Read the model definition and answer for the solid it produces. Units are mm, in the model's axes. Face numbers are marked on the shaded views. A direction names the side the tool comes from. Coordinates: 2 decimals unless noted, no trailing zeros. Order: outer loops, then holes, each group sorted by start corner. A loop starts at its lowest first (then second) coordinate and runs counter-clockwise, first axis right, second up. Notation, with made-up numbers: (10.5, -30.75) -> (54.5, -30.75) arc R20 cw to (54.5, -18.75) -> close; hole circle Ø5 at (17.5, 11). An arc over 180 degrees is marked (long way). Use CSV: the item, a comma, the result in double quotes.
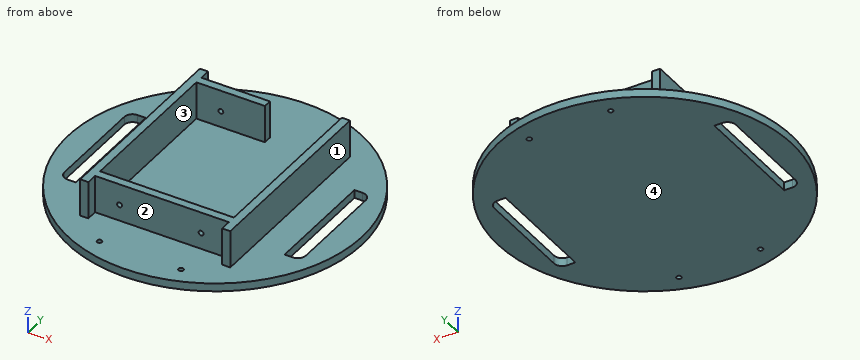
```python
from build123d import *

# Parameters (mm, degrees)
SKETCH_1_R          = 90
EXTRUDE_1_DEPTH     = 5
CUT_EXTRUDE_1_DEPTH = 128.377392029
SKETCH_2_R          = 1.5
CUT_EXTRUDE_2_DEPTH = 128.377392029
SKETCH_4_W          = 5
SKETCH_4_H          = 120
EXTRUDE_2_DEPTH     = 23
SKETCH_5_W          = 82
SKETCH_5_H          = 5
SKETCH_5_W_2        = 42
EXTRUDE_3_DEPTH     = 23
SKETCH_6_R          = 1.5
CUT_EXTRUDE_3_DEPTH = 172.477585999


with BuildPart() as part:
    # 草圖1 → 填料-伸長1 (new body)
    with BuildSketch(Plane.XY):
        Circle(SKETCH_1_R)
    extrude(amount=EXTRUDE_1_DEPTH)

    # 草圖3 → 除料-伸長1 (cut, through all)
    with BuildSketch(Plane.XY.offset(5)):
        with BuildLine():
            ThreePointArc((-69, -35), (-72.535533906, -33.535533906), (-74, -30))
            Line((-74, -30), (-74, 30))
            ThreePointArc((-74, 30), (-72.535533906, 33.535533906), (-69, 35))
            Line((-69, 35), (-64, 35))
            Line((-64, 35), (-64, -35))
            Line((-64, -35), (-69, -35))
        make_face()
        with BuildLine():
            Line((64, 35), (64, -35))
            Line((64, -35), (69, -35))
            ThreePointArc((69, -35), (72.535533906, -33.535533906), (74, -30))
            Line((74, -30), (74, 30))
            ThreePointArc((74, 30), (72.535533906, 33.535533906), (69, 35))
            Line((69, 35), (64, 35))
        make_face()
    extrude(amount=-CUT_EXTRUDE_1_DEPTH, mode=Mode.SUBTRACT)

    # 草圖2 → 除料-伸長2 (cut, through all)
    with BuildSketch(Plane.XY.offset(5)):
        with Locations((-25, 75)):
            Circle(SKETCH_2_R)
        with Locations(Location((-25, -75, 0), (0, 0, 180))):
            Circle(SKETCH_2_R)
        with Locations(Location((25, 75, 0), (0, 0, 180))):
            Circle(SKETCH_2_R)
        with Locations((25, -75)):
            Circle(SKETCH_2_R)
    extrude(amount=-CUT_EXTRUDE_2_DEPTH, mode=Mode.SUBTRACT)

    # 草圖4 → 填料-伸長2 (add)
    with BuildSketch(Plane.XY.offset(5)):
        with Locations((-43.5, 0)):
            Rectangle(SKETCH_4_W, SKETCH_4_H)
        with Locations((43.5, 0)):
            Rectangle(SKETCH_4_W, SKETCH_4_H)
    extrude(amount=EXTRUDE_2_DEPTH)

    # 草圖5 → 填料-伸長3 (add)
    with BuildSketch(Plane.XY.offset(5)):
        with Locations((0, -50.75)):
            Rectangle(SKETCH_5_W, SKETCH_5_H)
        with Locations((-20, 50.75)):
            Rectangle(SKETCH_5_W_2, SKETCH_5_H)
    extrude(amount=EXTRUDE_3_DEPTH)

    # 草圖6 → 除料-伸長3 (cut, through all)
    with BuildSketch(Plane(origin=(0, -53.25, 0), x_dir=(-1, 0, 0), z_dir=(0, -1, 0))):
        with Locations(Location((26, -15, 0), (0, 0, 90))):
            Circle(SKETCH_6_R)
        with Locations(Location((-24, -15, 0), (0, 0, 180))):
            Circle(SKETCH_6_R)
    extrude(amount=-CUT_EXTRUDE_3_DEPTH, mode=Mode.SUBTRACT)


solid = part.part
```
Item 1: Find section D-D, the plane x = -54. Give the vertices of the cut face in (y, z).
Return value:
outline,"(-72, 0) -> (72, 0) -> (72, 5) -> (-72, 5) -> close"
Item 2: A tool of negligible diameter and unlimited length cuts with its end or side. For the marked faces 1, 2, 3 and 4, from which of +Z, -Z, +X, -X, +Y, -Y can it reach the whole face along a straight path? Write none if from no direction.
Return value:
face 1,"+Z, +X, +Y, -Y"
face 2,"+Z, -Y"
face 3,"+Z"
face 4,"-Z, +X, -X, +Y, -Y"
Item 3: Straight lines are drawn through the part: line 1 along X through (y, z) = (51.9, 15); line 2 along X through (y, z) = (47.5, 26.75); line 3 along X through (y, z) = (4, 2). For each, find the intervals that lie inside material, in ascending order.
Return value:
line 1,"x = -46 to -27.5, -24.5 to 1, 41 to 46"
line 2,"x = -46 to -41, 41 to 46"
line 3,"x = -89.91 to -74, -64 to 64, 74 to 89.91"
Item 4: Find section A-A, the plane y = 0. Give the vertices of the cut face in (x, z), then the cut area to 3 significant figures.
Return value:
outline,"(-90, 0) -> (-74, 0) -> (-74, 5) -> (-90, 5) -> close; (-64, 0) -> (64, 0) -> (64, 5) -> (46, 5) -> (46, 28) -> (41, 28) -> (41, 5) -> (-41, 5) -> (-41, 28) -> (-46, 28) -> (-46, 5) -> (-64, 5) -> close; (74, 0) -> (90, 0) -> (90, 5) -> (74, 5) -> close"
area,"1,030 mm^2"
Item 5: Each of these flat-tipped pins is pushed along its axis until it touches: P1, Ø2.5, axis at x = 43.5, z = 21, coming from the +Y side; P2, Ø1.5, axis at x = 8.5, z = 21, coming from the -Y side; P3, Ø10, axis at x = -55.5, y = 40, coming from the -Z side; P4, Ø1, axis at x = 42.5, z = 24.5, coming from the -Y side. Where does it stop, or does it pass through?
Return value:
P1,"stops at y = 60"
P2,"stops at y = -53.25"
P3,"stops at z = 0"
P4,"stops at y = -60"
Item 6: Find section C-C, the plane x = -6. Give the vertices of the cut face in (y, z), then the cut area to 3 significant figures.
Return value:
outline,"(-89.8, 0) -> (89.8, 0) -> (89.8, 5) -> (53.25, 5) -> (53.25, 28) -> (48.25, 28) -> (48.25, 5) -> (-48.25, 5) -> (-48.25, 28) -> (-53.25, 28) -> (-53.25, 5) -> (-89.8, 5) -> close"
area,"1,130 mm^2"
Item 7: Find section B-B, the plane z = 19.75. Give the vertices of the cut face in (x, y), then the cut area to 3 significant figures.
Return value:
outline,"(-46, -60) -> (-41, -60) -> (-41, -53.25) -> (41, -53.25) -> (41, -60) -> (46, -60) -> (46, 60) -> (41, 60) -> (41, -48.25) -> (-41, -48.25) -> (-41, 48.25) -> (1, 48.25) -> (1, 53.25) -> (-41, 53.25) -> (-41, 60) -> (-46, 60) -> close"
area,"1,820 mm^2"
